Build history of the part. All positions in model axes, mm. A direction names the side the tool comes from. Give positions to 0.01 mm unless a question says otherwise; leave off trailing zeros. Order: outer loops, then holes, each group sorted by start corner. A loop starts at its lowest first (then second) coordinate and runs counter-clockwise, first axis right, second up. Notation, with made-up numbers: M 40.25,-30 L 90.25,-30 A14 cw 90.25,-12 Z; hole C 43.5,72.25 d10. An arc over 180 degrees is marked long. One line per item, written item: value.
from build123d import *

# Parameters (mm, degrees)
BOSS_EXTRUDE1_DEPTH     = 1
BOSS_EXTRUDE2_DEPTH     = 1.6
CUT_EXTRUDE1_DEPTH      = 18.397844694
CUT_EXTRUDE1_DEPTH_BACK = 18.397844694
SKETCH2_R               = 0.9


with BuildPart() as part:
    # Sketch1 → Boss-Extrude1 (new body)
    with BuildSketch(Plane(origin=(0, 0, 0), x_dir=(1, 0, 0), z_dir=(0, 1, 0))):
        with BuildLine():
            Line((-0.75, 10.875), (-0.75, 12.227019261))
            ThreePointArc((-0.75, 12.227019261), (-6.131762108, 10.604904217), (-10.22252415, 6.75))
            Line((-10.22252415, 6.75), (-8.975, 6.75))
            Line((-8.975, 6.75), (-8.975, 5.25))
            Line((-8.975, 5.25), (-11.067971811, 5.25))
            ThreePointArc((-11.067971811, 5.25), (-12.238613585, 0.52805067), (-11.479034226, -4.277180525))
            Line((-11.479034226, -4.277180525), (-10.251454559, -4.277180525))
            Line((-10.251454559, -4.277180525), (-10.261976171, -6.689868838))
            ThreePointArc((-10.261976171, -6.689868838), (5.21925282, -11.08250423), (11.693587987, 3.65))
            Line((11.693587987, 3.65), (9.875, 3.65))
            Line((9.875, 3.65), (9.875, 5.15))
            Line((9.875, 5.15), (11.114854925, 5.15))
            ThreePointArc((11.114854925, 5.15), (6.90758612, 10.116706678), (0.75, 12.227019261))
            Line((0.75, 12.227019261), (0.75, 10.875))
            Line((0.75, 10.875), (-0.75, 10.875))
        make_face()
    extrude(amount=BOSS_EXTRUDE1_DEPTH)

    # Sketch3 → Boss-Extrude2 (add)
    with BuildSketch(Plane(origin=(0, 1, 0), x_dir=(1, 0, 0), z_dir=(0, 1, 0))):
        with BuildLine():
            Line((-7.400720069, 2.725276386), (-7.400720069, -0.962016711))
            ThreePointArc((-7.400720069, -0.962016711), (1.548263455, 3.848750237), (8, -4))
            ThreePointArc((8, -4), (1.548263455, -11.848750237), (-7.400720069, -7.037983289))
            Line((-7.400720069, -7.037983289), (-7.400720069, -9.761754067))
            ThreePointArc((-7.400720069, -9.761754067), (1.115373522, -12.19911644), (9.048261309, -8.2578125))
            ThreePointArc((9.048261309, -8.2578125), (9.759165259, -6.181442975), (10, -4))
            ThreePointArc((10, -4), (3.605051963, 5.32757205), (-7.400720069, 2.725276386))
        make_face()
    extrude(amount=BOSS_EXTRUDE2_DEPTH)

    # Sketch2 → Cut-Extrude1 (cut, two sides: drawn at the far end of the back side and taken through both)
    with BuildSketch(Plane(origin=(0, 1, 0), x_dir=(1, 0, 0), z_dir=(0, 1, 0)).offset(-CUT_EXTRUDE1_DEPTH_BACK)):
        with BuildLine():
            Line((-11.479034226, -4.277180525), (-9.747973362, -4.277180525))
            Line((-9.747973362, -4.277180525), (-9.747973362, 0.222819475))
            Line((-9.747973362, 0.222819475), (-12.247973362, 0.222819475))
            ThreePointArc((-12.247973362, 0.222819475), (-12.074983324, -2.063317167), (-11.479034226, -4.277180525))
        make_face()
        with BuildLine():
            ThreePointArc((-7.400720069, -7.037983289), (8, -4), (-7.400720069, -0.962016711))
            Line((-7.400720069, -0.962016711), (-8, -2))
            Line((-8, -2), (-8.5, -2))
            Line((-8.5, -2), (-8.5, -6))
            Line((-8.5, -6), (-8, -6))
            Line((-8, -6), (-7.400720069, -7.037983289))
        make_face()
        with Locations(Location((9.5, -4.1, 0), (0, 0, 270))):
            Circle(SKETCH2_R)
    extrude(amount=CUT_EXTRUDE1_DEPTH + CUT_EXTRUDE1_DEPTH_BACK, mode=Mode.SUBTRACT)


solid = part.part
1) Drill centre lines: probe 1 along X at (y, z) = (0.8, 4.1); probe 2 along Y at (x, z) = (-2.25, -9.25); probe 3 along Z at (x, y) = (0, 0.6) (3 decimals). Where is each one in solid material? Low to high. Write a range as from..to.
Check values:
probe 1: -9.75..-8.5, 8..8.6, 10.4..11.54
probe 2: 0..1
probe 3: -10.875..-4, 12..12.25
2) Tool access for faces 1 (the face through (10.5, 0.5, -5.15)), 2 (the face through (-0.75, 0.5, -11.5)), 3 (the face through (-8.5, 0.5, 4)): list every direction of +Z, -Z, +X, -X, +Y, -Y with a clear straight run to the whole face (end or side of a thin tool).
Check values:
face 1: +X, +Y, -Y
face 2: -Z, +Y, -Y
face 3: +Y, -Y
3) Saw through at C-C, the plane z = -1.25. Write the cut outline in (x, y), then the cut area to 3 significant figures.
Check values:
outline: M -12.19,0 L -6.04,0 L -6.04,2.6 L -7.4,2.6 L -7.4,1 L -12.19,1 Z; M 6.04,0 L 12.19,0 L 12.19,1 L 8.51,1 L 8.51,2.6 L 6.04,2.6 Z
area: 18.4 mm^2
4) Saw through at A-A, the plane x = 0. Write the cut outline in (y, z) (3 decimals).
Check values:
outline: M 0,-10.875 L 1,-10.875 L 1,-6 L 2.6,-6 L 2.6,-4 L 0,-4 Z; M 0,12 L 2.6,12 L 2.6,12.25 L 0,12.25 Z
5) Saw through at D-D, the plane x = 9.5. Write the cut outline in (y, z), then the cut area to 3 significant figures.
Check values:
outline: M 0,-7.73 L 1,-7.73 L 1,0.88 L 2.6,0.88 L 2.6,3.2 L 0,3.2 Z; M 0,5 L 2.6,5 L 2.6,7.12 L 1,7.12 L 1,7.73 L 0,7.73 Z
area: 20.8 mm^2
6) Saw through at B-B, the plane y = 0.35. Write the cut outline in (x, z) (3 decimals).
Check values:
outline: M -12.248,-0.223 A12.25 ccw -11.068,-5.25 L -8.975,-5.25 L -8.975,-6.75 L -10.223,-6.75 A12.25 ccw -0.75,-12.227 L -0.75,-10.875 L 0.75,-10.875 L 0.75,-12.227 A12.25 ccw 11.115,-5.15 L 9.875,-5.15 L 9.875,-3.65 L 11.694,-3.65 A12.25 ccw -10.262,6.69 L -10.251,4.277 L -9.748,4.277 L -9.748,-0.223 Z; hole M -8.5,2 L -8,2 L -7.401,0.962 A8 ccw long -7.401,7.038 L -8,6 L -8.5,6 Z; hole C 9.5,4.1 d1.8
7) Pin check, flat tips, straight feed: pin 1 (10 mm diameter, centred on x = 1.5, z = 10, fed in from -Y); pin 2 (0.8 mm diameter, centred on x = -11, y = 0.5, fed in from +Z); pin 3 (1.5 mm diameter, centred on x = -1, y = 2.5, fed in from -Z); pin 4 (0.8 mm diameter, centred on x = 11, y = 0.5, fed in from -Z). Stop position of each tip, or through.
Check values:
pin 1: y = 0
pin 2: z = -0.22
pin 3: z = -6
pin 4: z = -6.14
8) Mould opens along X. For faces 4 (the face through (9.65, 1.79, 6.63)), 5 (the face through (-11, 0.5, -0.223)), 6 (the face through (0.75, 0.5, -11.6)) say: released by +X, released by -X, zero draft, split by the parting line, or undercut.
Check values:
face 4: released by +X
face 5: zero draft
face 6: undercut
